Print and shaded views of the part. All mm, measured from the part's lowest x, y and z. A direction names the side the tool comes from. Round coordinates to 2 decimals unless told otherwise and drop trailing zeros. Order: outer loops, then holes, each group sorted by start corner. A loop starts at its lowest first (then second) coordinate and runs counter-clockwise, first axis right, second up. Notation, with made-up numbers: (7, 39.25) - (14, 39.25) arc R32 ccw to (14, 65.25) - close; hole circle Ø6 at (71, 42). An arc over 180 degrees is marked (long way). Return JSON: item names as keys, results as strings. Group by question number.
Item 1: Probe probe 1 along X at (y, z) = (18.44, 22.1) (1 decimal); probe 2 along Z at (x, y) = (10.25, 26); probe 3 along Z at (x, y) = (16.5, 22) (1 decimal). List the from-to ranges inside material, lowest first.
Item 2: Saw through at D-D on y = 18.5. State how many separate pieces and enclosed holes the cut face has, and give its area (3 significant figures).
Item 3: Drop flat-ended pins along their axis: pin 1 (1.1 mm diameter, centred on x = 2, y = 20.5, fed in from -Z); pin 2 (4 mm diameter, centred on x = 2.5, z = 20, fed in from +Y); pin 3 (1.1 mm diameter, centred on x = 20, y = 13, fed in from -Z); pin 4 (6 mm diameter, centred on x = 6.5, y = 21, fed in from -Z) (1 decimal). Give the stop position or say it passes through.
Item 4: Saw through at C-C on y = 10.5. List the corners of the cut face in (x, z) (1 decimal), and give its area (3 significant figures).
Item 5: Saw through at B-B on x = 11.5. List the corners of the cut face in (y, z) (1 decimal).
Item 6: Saw through at A-A on z = 11.5. List the corners of the cut face in (x, y) (1 decimal), and give its area (3 significant figures).
Item 7: Tool access for the marked faces 4 and 5: list every direction of +Z, -Z, +X, -X, +Y, -Y with a clear straight run to the whole face (end or side of a thin tool).
Item 8: Two-plate mould, pull along Y, no slides. Class the marked faces 1, 2 and 3: released by +Y, released by -Y, zero draft, split by the parting line, or undercut.
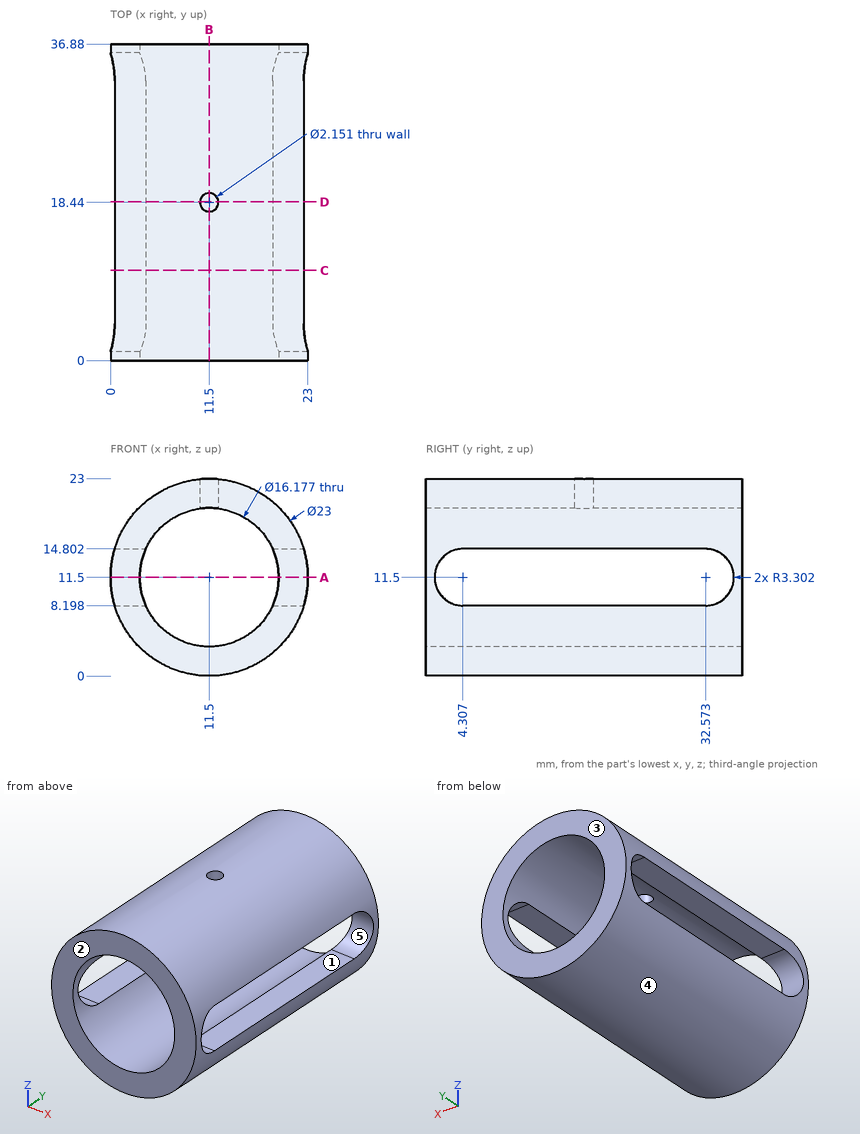
Filled in:
{
 "1": {"probe 1": "x = 7 to 10.4, 12.6 to 16", "probe 2": "z = 0.07 to 3.51, 19.49 to 22.93", "probe 3": "z = 1.1 to 5.1, 17.9 to 21.9"},
 "2": {"separate pieces": "3", "enclosed holes": "0", "area": "157 mm^2"},
 "3": {"pin 1": "stops at z = 4.28", "pin 2": "stops at y = 36.88", "pin 3": "stops at z = 3.19", "pin 4": "stops at z = 0.2"},
 "4": {"outline": "(0.5, 8.2) arc R11.5 ccw to (22.5, 8.2) - (18.9, 8.2) arc R8.1 cw to (4.1, 8.2) - close; (0.5, 14.8) - (4.1, 14.8) arc R8.1 cw to (18.9, 14.8) - (22.5, 14.8) arc R11.5 ccw to start", "area": "164 mm^2"},
 "5": {"outline": "(0, 0) - (36.9, 0) - (36.9, 3.4) - (0, 3.4) - close; (0, 19.6) - (17.4, 19.6) - (17.4, 23) - (0, 23) - close; (19.5, 19.6) - (36.9, 19.6) - (36.9, 23) - (19.5, 23) - close"},
 "6": {"outline": "(0, 0) - (3.4, 0) - (3.4, 1) - (0, 1) - close; (0, 35.9) - (3.4, 35.9) - (3.4, 36.9) - (0, 36.9) - close; (19.6, 0) - (23, 0) - (23, 1) - (19.6, 1) - close; (19.6, 35.9) - (23, 35.9) - (23, 36.9) - (19.6, 36.9) - close", "area": "13.7 mm^2"},
 "7": {"face 4": "+Y, -Y", "face 5": "+X, -X"},
 "8": {"face 1": "undercut", "face 2": "released by -Y", "face 3": "released by +Y"}
}
